Design review of the part built by this model. Coordinates are the model's own, in mm. A direction names the side the tool comes from. Round coordinates to 2 decimals unless told otherwise and drop trailing zeros. Order: outer loops, then holes, each group sorted by start corner. A loop starts at its lowest first (then second) coordinate and runs counter-clockwise, first axis right, second up. Notation, with made-up numbers: (78.25, 24.5) - (126.25, 24.5) arc R19 cw to (126.25, 33.5) - close; hole circle Ø2 at (-24.75, 54). An arc over 180 degrees is marked (long way). Use CSV: the item, a comma, the result in double quotes.
from build123d import *

# Parameters (mm, degrees)
SKETCH1_W           = 420
SKETCH1_H           = 127
BOSS_EXTRUDE1_DEPTH = 3
FILLET1_R           = 5
SKETCH2_R           = 1.5
CUT_EXTRUDE1_DEPTH  = 3
SKETCH3_W           = 144.6
SKETCH3_H           = 76.2
CUT_EXTRUDE2_DEPTH  = 3
FILLET2_R           = 10
SKETCH4_R           = 3.175
CUT_EXTRUDE3_DEPTH  = 10


with BuildPart() as part:
    # Sketch1 → Boss-Extrude1 (new body)
    with BuildSketch(Plane(origin=(0, 0, 0), x_dir=(1, 0, 0), z_dir=(0, 1, 0))):
        Rectangle(SKETCH1_W, SKETCH1_H)
    extrude(amount=BOSS_EXTRUDE1_DEPTH)

    # Fillet1
    fillet1_edges = [part.edges().sort_by_distance(p)[0] for p in [
        (210, 1.5, 63.5),
        (-210, 1.5, 63.5),
        (-210, 1.5, -63.5),
        (210, 1.5, -63.5),
    ]]
    fillet(fillet1_edges, radius=FILLET1_R)

    # Sketch2 → Cut-Extrude1 (cut)
    with BuildSketch(Plane(origin=(0, 3, 0), x_dir=(1, 0, 0), z_dir=(0, 1, 0))):
        with Locations(Location((200, -53.5, 0), (0, 0, 270))):
            Circle(SKETCH2_R)
        with Locations(Location((-200, -53.5, 0), (0, 0, 270))):
            Circle(SKETCH2_R)
        with Locations(Location((-200, 53.5, 0), (0, 0, 270))):
            Circle(SKETCH2_R)
        with Locations(Location((200, 53.5, 0), (0, 0, 270))):
            Circle(SKETCH2_R)
    extrude(amount=-CUT_EXTRUDE1_DEPTH, mode=Mode.SUBTRACT)

    # Sketch3 → Cut-Extrude2 (cut)
    with BuildSketch(Plane(origin=(0, 3, 0), x_dir=(1, 0, 0), z_dir=(0, 1, 0))):
        with Locations((112.3, 0)):
            Rectangle(SKETCH3_W, SKETCH3_H)
        with Locations((-112.3, 0)):
            Rectangle(SKETCH3_W, SKETCH3_H)
    extrude(amount=-CUT_EXTRUDE2_DEPTH, mode=Mode.SUBTRACT)

    # Fillet2
    fillet2_edges = [part.edges().sort_by_distance(p)[0] for p in [
        (-184.6, 1.5, -38.1),
        (-40, 1.5, -38.1),
        (-40, 1.5, 38.1),
        (-184.6, 1.5, 38.1),
        (184.6, 1.5, -38.1),
        (184.6, 1.5, 38.1),
        (40, 1.5, 38.1),
        (40, 1.5, -38.1),
    ]]
    fillet(fillet2_edges, radius=FILLET2_R)

    # Sketch4 → Cut-Extrude3 (cut)
    with BuildSketch(Plane(origin=(0, 3, 0), x_dir=(1, 0, 0), z_dir=(0, 1, 0))):
        with Locations(Location((0, 53.5, 0), (0, 0, 270))):
            Circle(SKETCH4_R)
        with Locations(Location((0, -53.5, 0), (0, 0, 270))):
            Circle(SKETCH4_R)
    extrude(amount=-CUT_EXTRUDE3_DEPTH, mode=Mode.SUBTRACT)


solid = part.part
1) We need section A-A (z = 5). Give the boundary of the cut face in (x, y).
Data:
outline,"(-210, 0) - (-184.6, 0) - (-184.6, 3) - (-210, 3) - close; (-40, 0) - (40, 0) - (40, 3) - (-40, 3) - close; (184.6, 0) - (210, 0) - (210, 3) - (184.6, 3) - close"
2) To check wall thickness, follow L1, parallel to X at y = 2.2, z = -3.5; L2, parallel to X at y = 1.75, z = 53.5 (3 decimals); L3, parallel to Z at x = -200, y = 0.8. State the ranges of each line that lie inside material, in increasing order. Write a range as from..to.
Data:
L1,"x = -210..-184.6, -40..40, 184.6..210"
L2,"x = -210..-201.5, -198.5..-3.175, 3.175..198.5, 201.5..210"
L3,"z = -63.5..-55, -52..52, 55..63.5"
3) For faces 3 (the face through (-3, 3, -1)), 4 (the face through (-43.01, 1.48, 35.25)), list the 3-axis set-ups (+Z, -Z, +X, -X, +Y, -Y) from which the entire face can be reached by the end or side of a thin tool; tool diameter is ignored.
Data:
face 3,"+Z, -Z, +X, -X, +Y"
face 4,"+Y, -Y"
4) We need section B-B (x = -100.5). Give the boundary of the cut face in (y, z).
Data:
outline,"(0, -63.5) - (3, -63.5) - (3, -38.1) - (0, -38.1) - close; (0, 38.1) - (3, 38.1) - (3, 63.5) - (0, 63.5) - close"
5) We need section C-C (y = 1.05). Give the number of separate pieces and of enclosed holes in the cut face, then the cut area to 3 significant figures.
Data:
separate pieces,"1"
enclosed holes,"8"
area,"31,400 mm2"
6) Insertion check: pin 1 Ø5 at (x, z) = (-68.5, -36) entering from +Y. The pin has a flat end and moves straight along its axis. Give the tip position at first contact, or say it passes through.
Data:
pin 1,"stops at y = 3"
7) The part is to be moulded in two halves that separate along Z. For faces 1 (the face through (-42.85, 1.48, -35.09)), 2 (the face through (-3, 0, -1)), say which applies: +Z half, -Z half, draft (parallel to the pull), parting line (faces both ways), or undercut.
Data:
face 1,"undercut"
face 2,"draft"
